Can you work these out from the model? Positions are in its coordinate system, mm. Face numbers are marked on the shaded views. Coordinates: 2 decimals unless noted, no trailing zeros. Order: outer loops, then holes, each group sorted by start corner. A loop starts at its lowest first (then second) coordinate and runs counter-clockwise, first axis right, second up. Notation, with made-up numbers: (-25.75, -10) -> (-0.75, -10) arc R29 ccw to (-0.75, 21) -> close; hole circle Ø7 at (54, 2). An arc over 180 degrees is marked (long way). Write item = value, one per line.
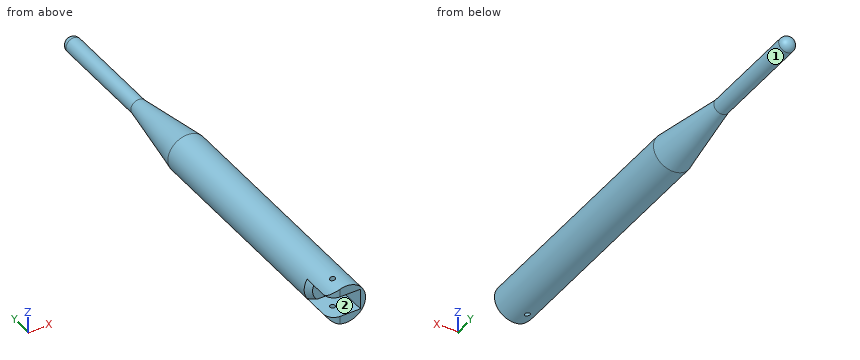
```python
from build123d import *

# Parameters (mm, degrees)
SKETCH3_R               = 7.5
BOSS_EXTRUDE1_DEPTH     = 18
CUT_EXTRUDE1_START      = -12
CUT_EXTRUDE1_DEPTH      = 12
CHAMFER1_SIZE           = 2
CUT_EXTRUDE2_DEPTH      = 92.041199465
CUT_EXTRUDE2_DEPTH_BACK = 92.041199465
CUT_EXTRUDE3_DEPTH      = 92.041199585
CUT_EXTRUDE3_DEPTH_BACK = 92.041199585
SKETCH7_R               = 1


with BuildPart() as part:
    # Sketch2 → Revolve1 (revolve)
    with BuildSketch(Plane.XY, mode=Mode.PRIVATE) as revolve1_sk:
        with BuildLine():
            Line((7.5, -72), (7.5, 8))
            Line((7.5, 8), (3, 38))
            Line((3, 38), (3, 78))
            ThreePointArc((3, 78), (2.121320344, 80.121320344), (0, 81))
            Line((0, 81), (0, -72))
            Line((0, -72), (7.5, -72))
        make_face()
    revolve(revolve1_sk.sketch.rotate(Axis((0, 81, 0), (0, -1, 0)), 90), axis=Axis((0, 81, 0), (0, -1, 0)))

    # Sketch3 → Boss-Extrude1 (add)
    with BuildSketch(Plane.XZ.offset(72)):
        with Locations(Location((0, 0, 0), (0, 0, 90))):
            Circle(SKETCH3_R)
    extrude(amount=BOSS_EXTRUDE1_DEPTH)

    # Sketch4 → Cut-Extrude1 (cut)
    with BuildSketch(Plane.XZ.offset(90).offset(CUT_EXTRUDE1_START)):
        with BuildLine():
            Line((5.5, 4), (-6.34428877, 4))
            ThreePointArc((-6.34428877, 4), (-7.5, 0), (-6.34428877, -4))
            Line((-6.34428877, -4), (5.5, -4))
            Line((5.5, -4), (5.5, -0.585443259))
            Line((5.5, -0.585443259), (5.5, 0.585443259))
            Line((5.5, 0.585443259), (5.5, 4))
        make_face()
    extrude(amount=CUT_EXTRUDE1_DEPTH, mode=Mode.SUBTRACT)

    # Chamfer1
    chamfer1_edges = [part.edges().sort_by_distance(p)[0] for p in [
        (-7.5, -78, 0),
    ]]
    chamfer(chamfer1_edges, length=CHAMFER1_SIZE)

    # Sketch6 → Cut-Extrude2 (cut, two sides: drawn at the far end of the back side and taken through both)
    with BuildSketch(Plane.XY.offset(-4).offset(-CUT_EXTRUDE2_DEPTH_BACK)):
        with BuildLine():
            Line((-6.34428877, -86), (-6.34428877, -90))
            Line((-6.34428877, -90), (-2.34428877, -90))
            ThreePointArc((-2.34428877, -90), (-5.172715895, -88.828427125), (-6.34428877, -86))
        make_face()
    extrude(amount=CUT_EXTRUDE2_DEPTH + CUT_EXTRUDE2_DEPTH_BACK, mode=Mode.SUBTRACT)

    # Sketch7 → Cut-Extrude3 (cut, two sides: drawn at the far end of the back side and taken through both)
    with BuildSketch(Plane.XY.offset(-4).offset(-CUT_EXTRUDE3_DEPTH_BACK)):
        with Locations((-1.5, -84)):
            Circle(SKETCH7_R)
    extrude(amount=CUT_EXTRUDE3_DEPTH + CUT_EXTRUDE3_DEPTH_BACK, mode=Mode.SUBTRACT)


solid = part.part
```
Item 1: If we mould it in two halves opening along Z, with no side actions, what happens to the marked faces 1 and 2? For each: pulls with the +Z half, pulls with the -Z half, needs draft (parallel to the pull), parting line crosses it, or undercut.
A:
face_1 = parting line crosses it
face_2 = undercut
Item 2: I want a section at C-C, the plane y = 43.5. Please give me the cut outline in (x, z), plus the area to 3 significant figures.
A:
outline = circle Ø6 at (0, 0)
area = 28.3 mm2
Item 3: I want a section at B-B, the plane y = -70. Please give me the cut outline in (x, z), plus the area to 3 significant figures.
A:
outline = circle Ø15 at (0, 0)
area = 177 mm2
Item 4: If I drill on probe 1 along X at (y, z) = (-84, -6.35); probe 2 along X at (y, z) = (-84, 5.9); probe 3 along Z at (x, y) = (-5.5, -80.5), over which ranges is the centre line in solid material (lowest first)?
A:
probe_1 = -3.99 to -2.5, -0.5 to 3.99
probe_2 = -4.63 to -2.5, -0.5 to 4.63
probe_3 = -5.1 to -4, 4 to 5.1
Item 5: I want a section at A-A, the plane z = 0. Please give me the cut outline in (x, y), plus the area to 3 significant figures.
A:
outline = (-7.5, -76) -> (-5.5, -78) -> (5.5, -78) -> (5.5, -90) -> (7.5, -90) -> (7.5, 8) -> (3, 38) -> (3, 78) arc R3 ccw to (-3, 78) -> (-3, 38) -> (-7.5, 8) -> close
area = 1,880 mm2
Item 6: I'm going to push flat-ended pins straight in: P1, Ø1, axis at x = -0.5, y = 37.5, coming from the -Z side; P2, Ø1.5, axis at y = -26.5, z = 5, coming from the +X side; P3, Ø1.2, axis at x = -1.5, y = -84, coming from the +Z side; P4, Ø8, axis at x = -1, y = 5.5, coming from the +Z side. Where does each tip first touch, or does it pass through?
A:
P1 = -3.13
P2 = 6.18
P3 = through
P4 = 7.5
